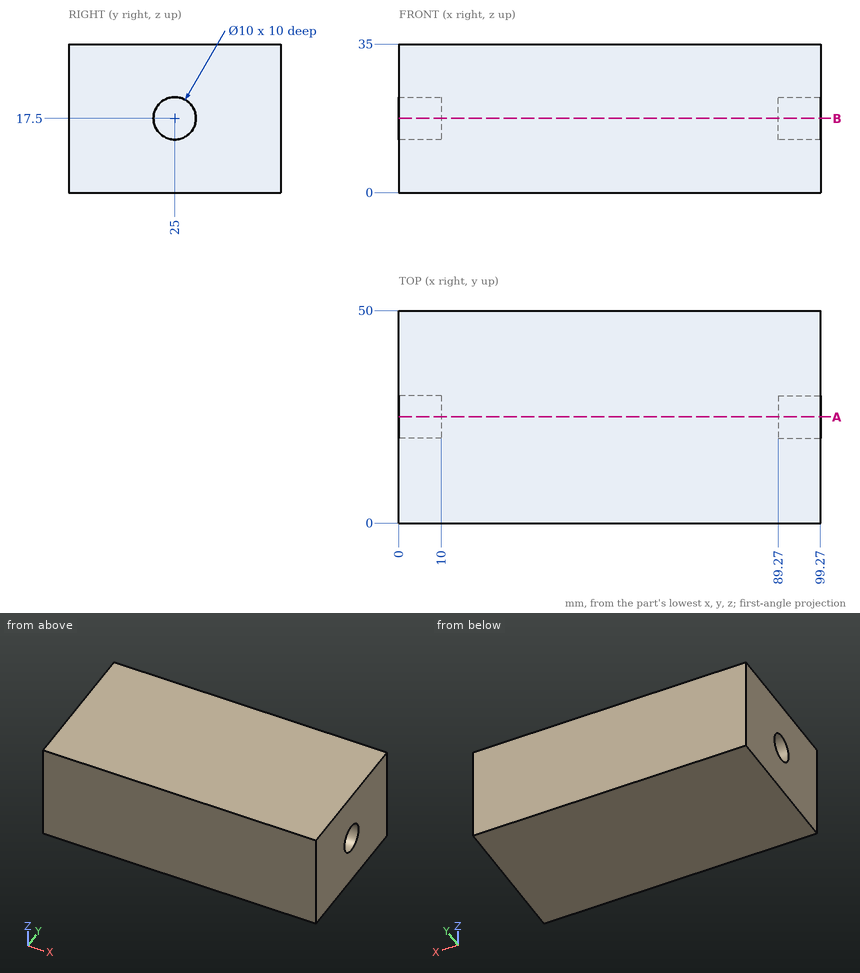
Design review of the part shown in the three views and the two pictorial views. Dimensions are in mm from the part's minimum x, y and z. Round coordinates to 2 decimals unless told otherwise and drop trailing zeros. Loops run counter-clockwise (first coordinate to the right, second up) from the corner with the lowest first, then second, coordinate; pieces in that order, holes last.
Q1. Add section A-A on y = 25. Write out the cut boundary in (x, z).
Result sheet:
outline: (0, 0) - (99.27, 0) - (99.27, 12.5) - (89.27, 12.5) - (89.27, 22.5) - (99.27, 22.5) - (99.27, 35) - (0, 35) - (0, 22.5) - (10, 22.5) - (10, 12.5) - (0, 12.5) - close
Q2. Insertion check: pin 1 Ø3 at (y, z) = (25.5, 19.5) entering from +X; pin 2 Ø2 at (y, z) = (6.5, 6.5) entering from -X; pin 3 Ø6 at (y, z) = (25, 17.5) entering from -X. Each pin has a flat end and moves straight along its axis. Give the tip position at first contact, or say it passes through.
Result sheet:
pin 1: stops at x = 89.27
pin 2: stops at x = 0
pin 3: stops at x = 10
Q3. To check wall thickness, follow line 1 along Y through (x, z) = (95.75, 17.5); line 2 along X through (y, z) = (25.5, 18). State the ranges of each line that lie inside material, in increasing order.
Result sheet:
line 1: y = 0 to 20, 30 to 50
line 2: x = 10 to 89.27
Q4. Add section B-B on z = 17.5. Write out the cut boundary in (x, y), plus the area to 3 significant figures.
Result sheet:
outline: (0, 0) - (99.27, 0) - (99.27, 20) - (89.27, 20) - (89.27, 30) - (99.27, 30) - (99.27, 50) - (0, 50) - (0, 30) - (10, 30) - (10, 20) - (0, 20) - close
area: 4,760 mm2
